Source: CAD feature listing. Evaluate the final solid. Frame: model axes, mm. Face numbers are marked on the shaded views. A direction names the side the tool comes from. Give positions to 0.01 mm unless a question says otherwise; leave off trailing zeros. Loops run counter-clockwise (first coordinate to the right, second up) from the corner with the lowest first, then second, coordinate; pieces in that order, holes last.
```python
from build123d import *

# Parameters (mm, degrees)
ESBO_O1_R                = 3.5
RESSALTO_EXTRUS_O1_DEPTH = 10
ESBO_O2_R                = 3
CORTE_EXTRUS_O1_DEPTH    = 10


with BuildPart() as part:
    # Esboço1 → Ressalto-extrusão1 (new body)
    with BuildSketch(Plane.XY):
        with BuildLine():
            Line((16.477791125, 11.172502957), (9.316356929, 42.949783159))
            ThreePointArc((9.316356929, 42.949783159), (6.482723548, 50.189321152), (-0.680221872, 53.211340576))
            Line((-0.680221872, 53.211340576), (-13.900221872, 53.211340576))
            ThreePointArc((-13.900221872, 53.211340576), (-17.435755778, 51.746874482), (-18.900221872, 48.211340576))
            Line((-18.900221872, 48.211340576), (-18.900221872, 43.211340576))
            Line((-18.900221872, 43.211340576), (-9.19947784, 15.541635731))
            ThreePointArc((-9.19947784, 15.541635731), (-5.879873215, 2.214686326), (-8.553040247, -11.256821879))
            Line((-8.553040247, -11.256821879), (-18.900221872, -40.946499789))
            Line((-18.900221872, -40.946499789), (-18.900221872, -45.946499789))
            ThreePointArc((-18.900221872, -45.946499789), (-17.851927459, -49.009835055), (-15.146612691, -50.788659424))
            Line((-15.146612691, -50.788659424), (-13.900221872, -50.788659424))
            Line((-13.900221872, -50.788659424), (-0.680221872, -50.788659424))
            ThreePointArc((-0.680221872, -50.788659424), (6.39084594, -47.859727235), (9.319778128, -40.788659424))
            Line((9.319778128, -40.788659424), (16.477791125, -8.749821804))
            Line((16.477791125, -8.749821804), (6.477791125, -8.749821804))
            ThreePointArc((6.477791125, -8.749821804), (3.350782595, -7.096987172), (2.099778128, -3.788659424))
            Line((2.099778128, -3.788659424), (2.099778128, 6.209261385))
            ThreePointArc((2.099778128, 6.209261385), (3.564118149, 9.745530472), (7.099778128, 11.211340576))
            Line((7.099778128, 11.211340576), (16.477791125, 11.172502957))
        make_face()
        with Locations((-6.950221872, 41.211340576)):
            Circle(ESBO_O1_R, mode=Mode.SUBTRACT)
        with Locations(Location((-6.950221872, -38.788659424, 0), (0, 0, 180))):
            Circle(ESBO_O1_R, mode=Mode.SUBTRACT)
        Polygon((-7.240418913, 33.581340576), (4.209581087, 33.581340576), (6.808835229, 18.845396153), align=None, mode=Mode.SUBTRACT)
        Polygon((4.209581087, -31.158659424), (6.808835229, -16.422715), (-7.240418913, -31.158659424), align=None, mode=Mode.SUBTRACT)
    extrude(amount=RESSALTO_EXTRUS_O1_DEPTH)

    # Esboço2 → Corte-extrusão1 (cut)
    with BuildSketch(Plane(origin=(2.099778128, 0, 0), x_dir=(0, 0, -1), z_dir=(1, 0, 0))):
        with Locations(Location((-4.928277881, 1.02125064, 0), (0, 0, 90))):
            Circle(ESBO_O2_R)
    extrude(amount=-CORTE_EXTRUS_O1_DEPTH, mode=Mode.SUBTRACT)


solid = part.part
```
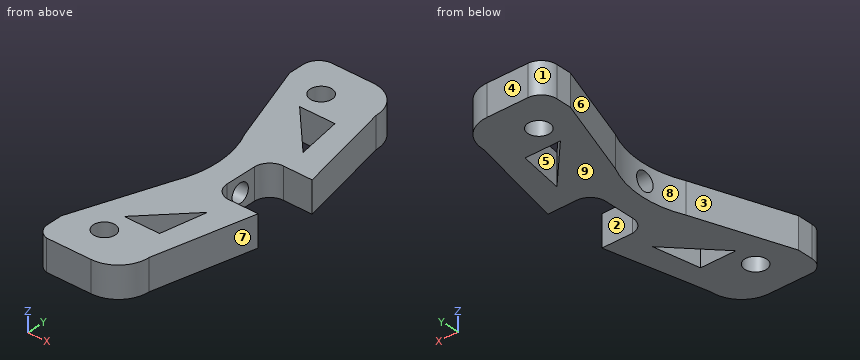
(1) First-contact query: pin 1 (6.5 mm diameter, centred on x = -6.95, y = -38.79, fed in from +Z); pin 2 (6 mm diameter, centred on y = 32, z = 5, fed in from +X); pin 3 (3 mm diameter, centred on x = 9, z = 2.5, fed in from -Y); pin 4 (4 mm diameter, centred on y = -18, z = 8.5, fed in from -X). Flat tips, straight axial feed; report the tip coordinate or a pass-through.
A:
pin 1: passes through
pin 2: stops at x = 12.46
pin 3: stops at y = -46.54
pin 4: stops at x = -11.6
(2) Mould query, pull axis Y, two halves, no side actions, for the marked faces 6, 7, 8 and 9. Classes: pulls with the +Y half, pulls with the -Y half, needs draft (parallel to the pull), parting line crosses it, or undercut.
A:
face 6: undercut
face 7: pulls with the -Y half
face 8: undercut
face 9: needs draft
(3) Reachability of the marked faces 1, 2, 3, 4 and 5 from +Z, -Z, +X, -X, +Y, -Y: full face, straight path, thin tool, end or side. Return the list, or none.
A:
face 1: +Z, -Z, -X, +Y
face 2: +Z, -Z, +X
face 3: +Z, -Z, -X
face 4: +Z, -Z, +X, -X, +Y
face 5: +Z, -Z
(4) Section D-D, the plane x = 10.5. Return the cut outline in (y, z).
A:
outline: (-35.51, 0) - (-8.75, 0) - (-8.75, 10) - (-35.51, 10) - close; (11.2, 0) - (37.7, 0) - (37.7, 10) - (11.2, 10) - close
(5) Section B-B, the plane y = 26.5. Return the cut outline in (x, z).
A:
outline: (-13.04, 0) - (-0.49, 0) - (-0.49, 10) - (-13.04, 10) - close; (5.46, 0) - (13.02, 0) - (13.02, 10) - (5.46, 10) - close
(6) Ray query, line 1 along Y through (x, z) = (-3, 9.25); line 2 along Y through (x, z) = (0, 4.5); line 3 along Y through (x, z) = (2.5, 8). Return the intervals inside material, ascending.
A:
line 1: y = -50.79 to -31.16, -26.71 to 29.13, 33.58 to 53.21
line 2: y = -50.77 to -31.16, -23.56 to -1.95, 3.99 to 25.99, 33.58 to 53.19
line 3: y = -50.27 to -31.16, -20.94 to -5.75, 8.17 to 23.36, 33.58 to 52.69
(7) Section A-A, the plane x = 0.5. Return the cut outline in (y, z), then the cut area to 3 significant figures.
A:
outline: (-50.72, 0) - (-31.16, 0) - (-31.16, 10) - (-50.72, 10) - close; (-23.04, 0) - (25.46, 0) - (25.46, 10) - (-23.04, 10) - close; (33.58, 0) - (53.14, 0) - (53.14, 10) - (33.58, 10) - close; hole circle Ø6 at (1.02, 4.93)
area: 848 mm2
(8) Section C-C, the plane z = 6.5. Count the separate pieces of the cut face and the enclosed holes in it, then the cut area to 3 significant figures.
A:
separate pieces: 2
enclosed holes: 4
area: 2,080 mm2
